Design review of the part built by this model. Coordinates are the model's own, in mm. A direction names the side the tool comes from. Coordinates: 2 decimals unless noted, no trailing zeros. Loops run counter-clockwise (first coordinate to the right, second up) from the corner with the lowest first, then second, coordinate; pieces in that order, holes last.
Q1. Add section C-C on y = 8.5. Give the boundary of the cut face in (x, z).
Q2. Add section B-B on z = 0. Give the boundary of the cut face in (x, y), and give its area (3 significant figures).
Q3. Machinability: for faces 1 (the face through (0, 27, 25.75)), 2 (the face through (2, 54, -26)), which of the approach directions +Z, -Z, +X, -X, +Y, -Y give a long, thin tool a straight path to every point of the face, cutting with its end or side? Answer none if there is none.
Q4. Draft analysis for pull direction X (two halves, no side actions). For faces 3 (the face through (27, 27, 0)), 4 (the face through (-27, 27, 0)), 5 (the face through (25.75, 27, 0)), 6 (the face through (0, 27, -27)), state which applies: released by +X, released by -X, zero draft, split by the parting line, or undercut.
Q5. Add section A-A on x = 12. Give the boundary of the cut face in (y, z), and give its area (3 significant figures).
Q6. For P1, Ø10, axis at x = -21.5, z = 5, coming from the -Y side, flat-tipped, find the tip position at first contact; note if it passes through.
Q7. Wall thickness on probe 1 along Z at (x, y) = (-9.5, 39): over which ranges is the line inside the solid? List them lowest first.
Autodesk Inventor part; units mm, degrees
ref_plane "YZ Plane" through (0, 0, 0) normal (1, 0, 0) x (0, 1, 0)
ref_plane "XZ Plane" through (0, 0, 0) normal (0, 1, 0) x (-1, 0, 0)
ref_plane "XY Plane" through (0, 0, 0) normal (0, 0, 1) x (1, 0, 0)
sketch "Sketch2" plane through (0, 0, 0) normal (0, 1, 0) x (-1, 0, 0)
  line L0 (27, 27) -> (-27, 27)
  line L1 (-27, 27) -> (-27, -27)
  line L2 (-27, -27) -> (27, -27)
  line L3 (27, -27) -> (27, 27)
  line L4 (27, 27) -> (-27, -27) construction
  line L5 (-27, 27) -> (27, -27) construction
  line L6 (25.75, -25.75) -> (-25.75, -25.75)
  line L7 (-25.75, -25.75) -> (-25.75, 25.75)
  line L8 (-25.75, 25.75) -> (25.75, 25.75)
  line L9 (25.75, 25.75) -> (25.75, -25.75)
  dimension "d31" = 54
  dimension "d32" = 54
  dimension "d43" = 1.25
extrude "Extrusion5" add sketch "Sketch2" along normal blind 54
properties part number "Cube" material "ABS Plastic"
Entries:
1. outline: (-27, -27) - (27, -27) - (27, 27) - (-27, 27) - close; hole (-25.75, -25.75) - (25.75, -25.75) - (25.75, 25.75) - (-25.75, 25.75) - close
2. outline: (-27, 0) - (-25.75, 0) - (-25.75, 54) - (-27, 54) - close; (25.75, 0) - (27, 0) - (27, 54) - (25.75, 54) - close
2. area: 135 mm2
3. face 1: +Y, -Y
3. face 2: +Z, -Z, +X, -X, +Y
4. face 3: released by +X
4. face 4: released by -X
4. face 5: undercut
4. face 6: zero draft
5. outline: (0, -27) - (54, -27) - (54, -25.75) - (0, -25.75) - close; (0, 25.75) - (54, 25.75) - (54, 27) - (0, 27) - close
5. area: 135 mm2
6. P1: stops at y = 0
7. probe 1: z = -27 to -25.75, 25.75 to 27
